Read the model definition and answer for the solid it produces. Units are mm, in the model's axes. Face numbers are marked on the shaded views. Round coordinates to 2 decimals unless told otherwise and drop trailing zeros. Put each result on its own line as item: value.
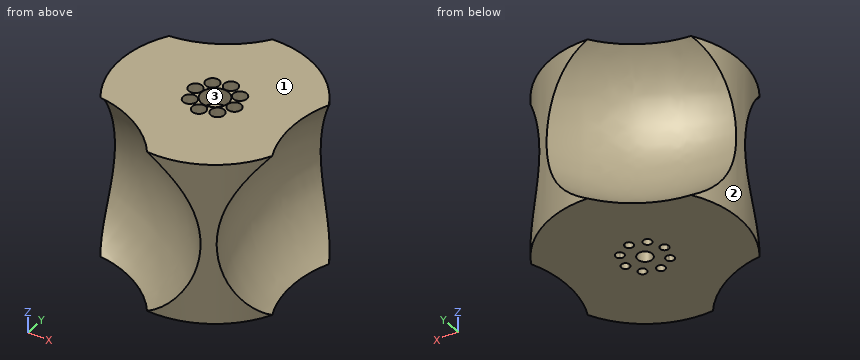
from build123d import *

# Parameters (mm, degrees)
F0_R          = 44.45
F0_R_2        = 16.51
F1_DEPTH      = 38.1
F1_DEPTH_BACK = 38.1
F4_R          = 3.175
F4_R_2        = 1.9685
F5_DEPTH      = 48.26
F6_R          = 6.35
F7_DEPTH      = 7.62
F8_R          = 3.429
F9_DEPTH      = 68.58


with BuildPart() as f1:
    # F0 (on Top) → F1 (new body, two sides)
    with BuildSketch(Plane.XY) as f1_sk:
        with Locations((-96.7949852347, 47.625)):
            Circle(F0_R)
        with Locations((-96.7949852347, 47.625)):
            Circle(F0_R_2, mode=Mode.SUBTRACT)
        with Locations((-96.7949852347, 47.625)):
            Circle(F0_R_2)
        with BuildLine():
            ThreePointArc((-88.1051627648, 52.1100670498), (-87.4115771175, 50.37826953), (-87.0594782396, 48.5462733292))
            ThreePointArc((-87.0594782396, 48.5462733292), (-85.6757800173, 47.965243489), (-85.103715896, 46.5778145407))
            ThreePointArc((-85.103715896, 46.5778145407), (-85.8323827306, 45.0488259953), (-87.478931514, 44.6517889292))
            ThreePointArc((-87.478931514, 44.6517889292), (-88.2130581693, 42.9367840447), (-89.2595036018, 41.3923956038))
            ThreePointArc((-89.2595036018, 41.3923956038), (-88.839336444, 40.7569162622), (-88.6919210429, 40.0094919292))
            ThreePointArc((-88.6919210429, 40.0094919292), (-90.1000831422, 38.1224270954), (-92.309918185, 38.9351775301))
            ThreePointArc((-92.309918185, 38.9351775301), (-94.0417157047, 38.2415918827), (-95.8737119056, 37.8894930048))
            ThreePointArc((-95.8737119056, 37.8894930048), (-98.0529677671, 35.9450498204), (-99.7681963056, 38.3089462792))
            ThreePointArc((-99.7681963056, 38.3089462792), (-101.48320119, 39.0430729345), (-103.0275896309, 40.089518367))
            ThreePointArc((-103.0275896309, 40.089518367), (-105.9434851899, 40.2555560033), (-105.4848077047, 43.1399329502))
            ThreePointArc((-105.4848077047, 43.1399329502), (-106.178393352, 44.87173047), (-106.5304922299, 46.7037266708))
            ThreePointArc((-106.5304922299, 46.7037266708), (-108.4749354144, 48.8829825323), (-106.1110389555, 50.5982110708))
            ThreePointArc((-106.1110389555, 50.5982110708), (-105.3769123002, 52.3132159553), (-104.3304668677, 53.8576043962))
            ThreePointArc((-104.3304668677, 53.8576043962), (-104.1644292314, 56.7734999551), (-101.2800522845, 56.3148224699))
            ThreePointArc((-101.2800522845, 56.3148224699), (-99.5482547647, 57.0084081173), (-97.7162585639, 57.3605069952))
            ThreePointArc((-97.7162585639, 57.3605069952), (-95.7414309138, 59.3162590358), (-93.7792997754, 57.3477693387))
            ThreePointArc((-93.7792997754, 57.3477693387), (-93.7899471678, 57.1433056087), (-93.8217741639, 56.9410537208))
            ThreePointArc((-93.8217741639, 56.9410537208), (-92.1067692795, 56.2069270655), (-90.5623808386, 55.160481633))
            ThreePointArc((-90.5623808386, 55.160481633), (-88.4202847093, 55.5757742752), (-87.210977164, 53.7595641919))
            ThreePointArc((-87.210977164, 53.7595641919), (-87.4489020941, 52.8214265806), (-88.1051627648, 52.1100670498))
        make_face(mode=Mode.SUBTRACT)
        with BuildLine():
            ThreePointArc((-87.478931514, 44.6517889292), (-89.0293967369, 46.7886116136), (-87.0594782396, 48.5462733292))
            ThreePointArc((-87.0594782396, 48.5462733292), (-87.4115771175, 50.37826953), (-88.1051627648, 52.1100670498))
            ThreePointArc((-88.1051627648, 52.1100670498), (-90.7124690483, 52.524684387), (-90.5623808386, 55.160481633))
            ThreePointArc((-90.5623808386, 55.160481633), (-92.1067692795, 56.2069270655), (-93.8217741639, 56.9410537208))
            ThreePointArc((-93.8217741639, 56.9410537208), (-95.9585968484, 55.3905884978), (-97.7162585639, 57.3605069952))
            ThreePointArc((-97.7162585639, 57.3605069952), (-99.5482547647, 57.0084081173), (-101.2800522845, 56.3148224699))
            ThreePointArc((-101.2800522845, 56.3148224699), (-101.0424845928, 55.8008459714), (-100.9610494266, 55.2405080708))
            ThreePointArc((-100.9610494266, 55.2405080708), (-102.1821250936, 53.4194234719), (-104.3304668677, 53.8576043962))
            ThreePointArc((-104.3304668677, 53.8576043962), (-105.3769123002, 52.3132159553), (-106.1110389555, 50.5982110708))
            ThreePointArc((-106.1110389555, 50.5982110708), (-104.988766028, 49.9120186247), (-104.5492545734, 48.6721854593))
            ThreePointArc((-104.5492545734, 48.6721854593), (-105.1303256251, 47.2757495806), (-106.5304922299, 46.7037266708))
            ThreePointArc((-106.5304922299, 46.7037266708), (-106.178393352, 44.87173047), (-105.4848077047, 43.1399329502))
            ThreePointArc((-105.4848077047, 43.1399329502), (-103.4723556943, 43.221010878), (-102.4419933055, 41.4904358081))
            ThreePointArc((-102.4419933055, 41.4904358081), (-102.5942832222, 40.7312433534), (-103.0275896309, 40.089518367))
            ThreePointArc((-103.0275896309, 40.089518367), (-101.48320119, 39.0430729345), (-99.7681963056, 38.3089462792))
            ThreePointArc((-99.7681963056, 38.3089462792), (-97.6377069641, 39.8600832689), (-95.8736706941, 37.9022306613))
            ThreePointArc((-95.8736706941, 37.9022306613), (-95.873680997, 37.8958617997), (-95.8737119056, 37.8894930048))
            ThreePointArc((-95.8737119056, 37.8894930048), (-94.0417157047, 38.2415918827), (-92.309918185, 38.9351775301))
            ThreePointArc((-92.309918185, 38.9351775301), (-91.8953008477, 41.5424838136), (-89.2595036018, 41.3923956038))
            ThreePointArc((-89.2595036018, 41.3923956038), (-88.2130581693, 42.9367840447), (-87.478931514, 44.6517889292))
        make_face()
    extrude(amount=F1_DEPTH)
    extrude(f1_sk.sketch, amount=-F1_DEPTH_BACK)

    # F2 (on Top) → F3 (revolve, cut)
    with BuildSketch(Plane.XY):
        with BuildLine():
            Line((-93.0453224617, -28.6843935659), (-128.9005062292, -7.9833935659))
            Line((-128.9005062292, -7.9833935659), (-175.7542126247, 19.0676064341))
            Line((-175.7542126247, 19.0676064341), (-194.8916419976, 30.1166064341))
            ThreePointArc((-194.8916419976, 30.1166064341), (-152.7765062292, -49.3378386474), (-62.9093704608, -46.0833935659))
            Line((-62.9093704608, -46.0833935659), (-93.0453224617, -28.6843935659))
        make_face()
        with BuildLine():
            Line((-164.7556899967, 82.5323935659), (-128.9005062292, 103.2333935659))
            Line((-128.9005062292, 103.2333935659), (-82.0467998336, 130.2843935659))
            Line((-82.0467998336, 130.2843935659), (-62.9093704608, 141.3333935659))
            ThreePointArc((-62.9093704608, 141.3333935659), (-152.7765062292, 144.5878386474), (-194.8916419976, 65.1333935659))
            Line((-194.8916419976, 65.1333935659), (-164.7556899967, 82.5323935659))
        make_face()
        with BuildLine():
            Line((-32.5839432458, 89.027), (-32.5839432458, 47.625))
            Line((-32.5839432458, 47.625), (-32.5839432458, -6.477))
            Line((-32.5839432458, -6.477), (-32.5839432458, -28.575))
            ThreePointArc((-32.5839432458, -28.575), (15.1680567542, 47.625), (-32.5839432458, 123.825))
            Line((-32.5839432458, 123.825), (-32.5839432458, 89.027))
        make_face()
    revolve(axis=Axis((-134.3997675432, -4.8083935659, 0), (0.8660254038, -0.5, 0)), mode=Mode.SUBTRACT)

    # F4 (on face) → F5 (cut)
    with BuildSketch(Plane.XY.offset(38.1)):
        with Locations((-102.9295494266, 55.2405080708)):
            Circle(F4_R)
        with Locations((-102.9295494266, 55.2405080708)):
            Circle(F4_R_2, mode=Mode.SUBTRACT)
        with Locations((-95.7477997754, 57.3477693387)):
            Circle(F4_R)
        with Locations((-95.7477997754, 57.3477693387)):
            Circle(F4_R_2, mode=Mode.SUBTRACT)
        with Locations((-89.179477164, 53.7595641919)):
            Circle(F4_R)
        with Locations((-89.179477164, 53.7595641919)):
            Circle(F4_R_2, mode=Mode.SUBTRACT)
        with Locations((-87.072215896, 46.5778145407)):
            Circle(F4_R)
        with Locations((-87.072215896, 46.5778145407)):
            Circle(F4_R_2, mode=Mode.SUBTRACT)
        with Locations((-90.6604210429, 40.0094919292)):
            Circle(F4_R)
        with Locations((-90.6604210429, 40.0094919292)):
            Circle(F4_R_2, mode=Mode.SUBTRACT)
        with Locations((-97.8421706941, 37.9022306613)):
            Circle(F4_R)
        with BuildLine():
            ThreePointArc((-95.8736706941, 37.9022306613), (-95.873680997, 37.8958617997), (-95.8737119056, 37.8894930048))
            ThreePointArc((-95.8737119056, 37.8894930048), (-99.8106603912, 37.9085995228), (-95.8736706941, 37.9022306613))
        make_face(mode=Mode.SUBTRACT)
        with Locations((-104.4104933055, 41.4904358081)):
            Circle(F4_R)
        with Locations((-104.4104933055, 41.4904358081)):
            Circle(F4_R_2, mode=Mode.SUBTRACT)
        with Locations((-106.5177545734, 48.6721854593)):
            Circle(F4_R)
        with Locations((-106.5177545734, 48.6721854593)):
            Circle(F4_R_2, mode=Mode.SUBTRACT)
    extrude(amount=-F5_DEPTH, mode=Mode.SUBTRACT)

    # F6 (on face) → F7 (cut)
    with BuildSketch(Plane.XY.offset(38.1)):
        with Locations((-96.7949852347, 47.625)):
            Circle(F6_R)
    extrude(amount=-F7_DEPTH, mode=Mode.SUBTRACT)

    # F8 (on face) → F9 (cut, through all)
    with BuildSketch(Plane.XY.offset(30.48)):
        with Locations((-96.7949852347, 47.625)):
            Circle(F8_R)
    extrude(amount=-F9_DEPTH, mode=Mode.SUBTRACT)

    # F2 (on Top) → F10 (revolve, cut)
    with BuildSketch(Plane.XY):
        with BuildLine():
            Line((-32.5839432458, 89.027), (-32.5839432458, 47.625))
            Line((-32.5839432458, 47.625), (-32.5839432458, -6.477))
            Line((-32.5839432458, -6.477), (-32.5839432458, -28.575))
            ThreePointArc((-32.5839432458, -28.575), (15.1680567542, 47.625), (-32.5839432458, 123.825))
            Line((-32.5839432458, 123.825), (-32.5839432458, 89.027))
        make_face()
    revolve(axis=Axis((-32.5839432458, 85.725, 0), (0, 1, 0)), mode=Mode.SUBTRACT)

    # F2 (on Top) → F11 (revolve, cut)
    with BuildSketch(Plane.XY):
        with BuildLine():
            Line((-164.7556899967, 82.5323935659), (-128.9005062292, 103.2333935659))
            Line((-128.9005062292, 103.2333935659), (-82.0467998336, 130.2843935659))
            Line((-82.0467998336, 130.2843935659), (-62.9093704608, 141.3333935659))
            ThreePointArc((-62.9093704608, 141.3333935659), (-152.7765062292, 144.5878386474), (-194.8916419976, 65.1333935659))
            Line((-194.8916419976, 65.1333935659), (-164.7556899967, 82.5323935659))
        make_face()
    revolve(axis=Axis((-123.4012449152, 106.4083935659, 0), (-0.8660254038, -0.5, 0)), mode=Mode.SUBTRACT)


solid = f1.part
Item 1: For a pull along X with two mould halves and no side action, classify the marked faces 1, 2 and 3 as pulls with the +X half, pulls with the -X half, needs draft (parallel to the pull), parting line crosses it, or undercut.
Derived:
face 1: needs draft
face 2: pulls with the -X half
face 3: undercut
Item 2: Flat-ended cylindrical pins translate along their axes: pin 1 Ø2 at (y, z) = (62, -9) entering from -X; pin 2 Ø6 at (x, z) = (-119.5, 16) entering from +Y; pin 3 Ø5 at (y, z) = (56, 21.5) entering from -X (3 decimals). Find the tip coordinate at first contact, or state that the pin passes through.
Derived:
pin 1: stops at x = -108.44
pin 2: stops at y = 59.89
pin 3: stops at x = -140.855
Item 3: Find the intervals of material crossed by line 1 along Y through (x, z) = (-95.5, 33); line 2 along Y through (x, z) = (-102, 6.5); line 3 along X through (y, z) = (50, -9), in increasing order.
Derived:
line 1: y = 8.34 to 35.76, 40.05 to 41.41, 53.84 to 54.18, 60.51 to 86.91
line 2: y = 31.01 to 39.42, 43.56 to 52.2, 58.28 to 64.24
line 3: x = -141.18 to -109.4, -103.63 to -99.27, -94.32 to -79.45
Item 4: The part is cut by section A-A (z = 16.5). State how many separate pieces and enclosed holes the cut face has, then the cut area to 3 significant figures.
Derived:
separate pieces: 1
enclosed holes: 9
area: 2,300 mm^2
